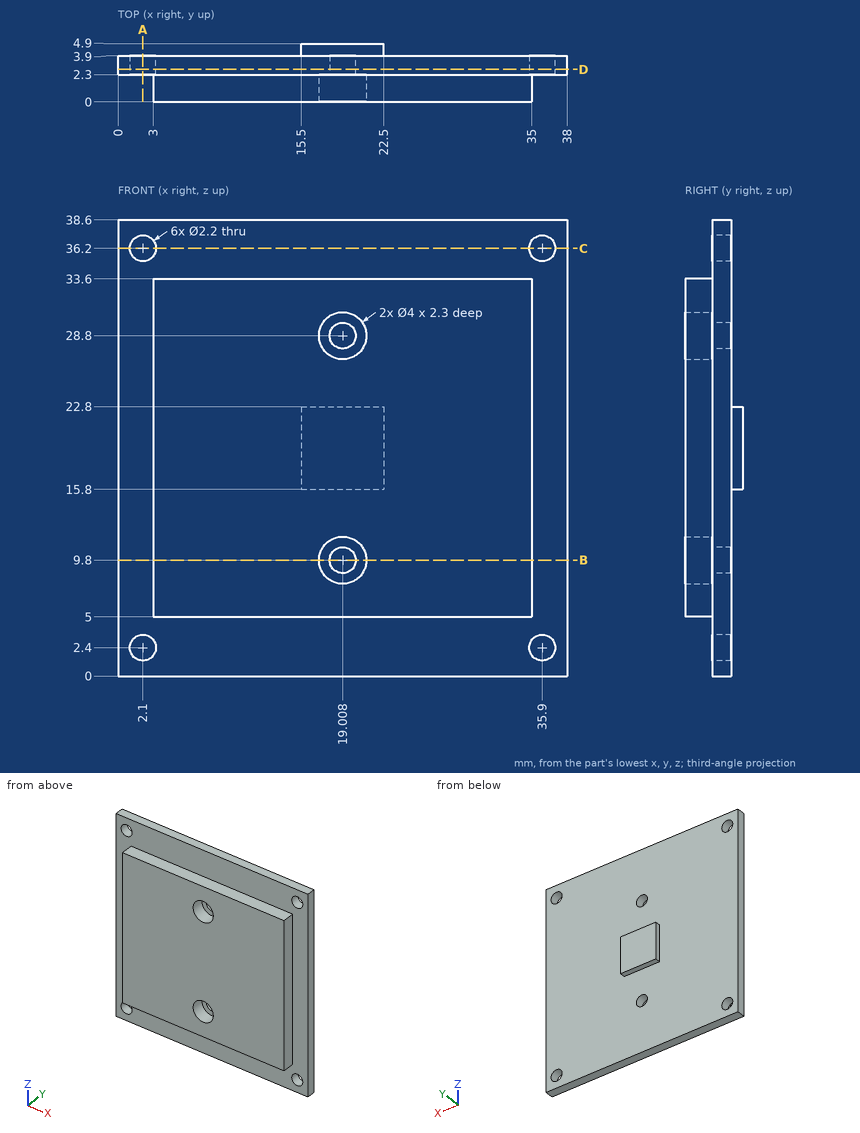
Print and shaded views of the part. All mm, measured from the part's lowest x, y and z. Round coordinates to 2 decimals unless told otherwise and drop trailing zeros. Write each loop counter-clockwise with the first axis right and the second up, starting at its lowest first coordinate (ties: lowest second). Pieces come first, ordered by that corner, then holes. Notation, with made-up numbers: (15, 26.25) -> (37, 26.25) arc R28 cw to (37, 58.25) -> close; hole circle Ø4 at (40.5, 28.25). An arc over 180 degrees is marked (long way). Return JSON: item names as keys, results as strings. Group by question number.
Q1. Saw through at C-C on z = 36.2. Write the cut outline in (x, y).
Q2. Pin check, flat tips, straight feed: pin 1 (3.5 mm diameter, centred on x = 19.01, z = 28.8, fed in from -Y); pin 2 (0.8 mm diameter, centred on x = 20, y = 4.5, fed in from +Z); pin 3 (0.7 mm diameter, centred on x = 26.5, y = 1.5, fed in from +Z). Stop position of each tip, or through.
Q3. Probe L1, parallel to X at y = 2.8, z = 36.2; L2, parallel to Z at x = 35.9, y = 3.3; L3, parallel to X at y = 3.25, z = 9.8. List the from-to ranges inside material, lowest first. Write a range as [from, to].
Q4. Saw through at B-B on z = 9.8. Write the cut outline in (x, y), plus the area to 3 significant figures.
Q5. Saw through at D-D on y = 2.75. Write the cut outline in (x, z), plus the area to 3 significant figures.
Q6. Saw through at A-A on x = 2.1. Write the cut outline in (y, z), plus the area to 3 significant figures.
Answer:
{
 "1": {"outline": "(0, 2.3) -> (1, 2.3) -> (1, 3.9) -> (0, 3.9) -> close; (3.2, 2.3) -> (34.8, 2.3) -> (34.8, 3.9) -> (3.2, 3.9) -> close; (37, 2.3) -> (38, 2.3) -> (38, 3.9) -> (37, 3.9) -> close"},
 "2": {"pin 1": "y = 2.3", "pin 2": "z = 22.8", "pin 3": "z = 33.6"},
 "3": {"L1": "[0, 1], [3.2, 34.8], [37, 38]", "L2": "[0, 1.3], [3.5, 35.1], [37.3, 38.6]", "L3": "[0, 17.91], [20.11, 38]"},
 "4": {"outline": "(0, 2.3) -> (3, 2.3) -> (3, 0) -> (17.01, 0) -> (17.01, 2.3) -> (17.91, 2.3) -> (17.91, 3.9) -> (0, 3.9) -> close; (20.11, 2.3) -> (21.01, 2.3) -> (21.01, 0) -> (35, 0) -> (35, 2.3) -> (38, 2.3) -> (38, 3.9) -> (20.11, 3.9) -> close", "area": "122 mm2"},
 "5": {"outline": "(0, 0) -> (38, 0) -> (38, 38.6) -> (0, 38.6) -> close; hole circle Ø2.2 at (2.1, 2.4); hole circle Ø2.2 at (2.1, 36.2); hole circle Ø2.2 at (19.01, 9.8); hole circle Ø2.2 at (19.01, 28.8); hole circle Ø2.2 at (35.9, 2.4); hole circle Ø2.2 at (35.9, 36.2)", "area": "1,440 mm2"},
 "6": {"outline": "(2.3, 0) -> (3.9, 0) -> (3.9, 1.3) -> (2.3, 1.3) -> close; (2.3, 3.5) -> (3.9, 3.5) -> (3.9, 35.1) -> (2.3, 35.1) -> close; (2.3, 37.3) -> (3.9, 37.3) -> (3.9, 38.6) -> (2.3, 38.6) -> close", "area": "54.7 mm2"}
}
